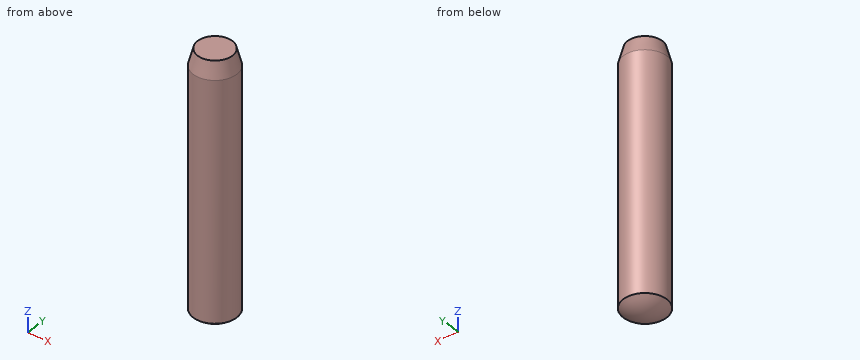
```python
from build123d import *

# Parameters (mm, degrees)
CROQUIS1_R              = 2
SALIENTE_EXTRUIR1_DEPTH = 24
CHAFL_N1_SIZE           = 1.5
CHAFL_N1_SIZE2          = 0.4


with BuildPart() as part:
    # Croquis1 → Saliente-Extruir1 (new body)
    with BuildSketch(Plane.XY):
        Circle(CROQUIS1_R)
    extrude(amount=SALIENTE_EXTRUIR1_DEPTH)

    # Croquis2 → Cortar-Revolución3 (revolve, cut)
    with BuildSketch(Plane(origin=(0, 0, 0), x_dir=(1, 0, 0), z_dir=(0, 1, 0))):
        with BuildLine():
            Line((-2, -0.75), (-2, 0))
            Line((-2, 0), (-2, 0.2))
            Line((-2, 0.2), (0, 0.2))
            Line((0, 0.2), (0, 0))
            ThreePointArc((0, 0), (-1.068000468, -0.193665418), (-2, -0.75))
        make_face()
    revolve(axis=Axis((0, 0, 24), (0, 0, -1)), mode=Mode.SUBTRACT)

    # Chaflán1
    chafl_n1_edges = [part.edges().sort_by_distance(p)[0] for p in [
        (-2, 0, 24),
    ]]
    chafl_n1_side = [part.faces().sort_by_distance(p)[0] for p in [
        (-2, 0, 12.375),
    ]]
    chamfer(chafl_n1_edges, length=CHAFL_N1_SIZE, length2=CHAFL_N1_SIZE2, reference=chafl_n1_side[0])


solid = part.part
```
Verification items for the finished model (mm, model axes). Round coordinates to 2 decimals unless told otherwise and drop trailing zeros. Write each loop counter-clockwise with the first axis right and the second up, starting at its lowest first coordinate (ties: lowest second). Pieces come first, ordered by that corner, then holes. Notation, with made-up numbers: (88.5, -34) -> (126.5, -34) arc R16 cw to (126.5, -5) -> close; hole circle Ø10 at (-14.75, 75). An arc over 180 degrees is marked (long way). Write each question's results on one line, items separated by ' | '. Start each with the question number.
1. Material ranges on probe 1 along Z at (x, y) = (-0.05, 0.05); probe 2 along X at (y, z) = (-1.45, 8.25); probe 3 along X at (y, z) = (-0.3, 3.5), recorded low to high. Write a range as from..to.
2. Depth check by flat-ended pin: P1, Ø2, axis at y = -1, z = 17.5, coming from the -X side; P2, Ø1.5, axis at x = -1, y = 0, coming from the -Z side. Enter the tip coordinate at first touch or a pass-through.
3. Cross-section at A-A (y = 0). Enter the section's corners in (x, z), then the cut area to 3 significant figures.
4. Cross-section at C-C (z = 10). Enter the section's corners in (x, y).
Solutions:
1) probe 1: z = 0..24 | probe 2: x = -1.38..1.38 | probe 3: x = -1.98..1.98
2) P1: stops at x = -2 | P2: stops at z = 0.01
3) outline: (-2, 0.75) arc R3.04 ccw to (2, 0.75) -> (2, 22.5) -> (1.6, 24) -> (-1.6, 24) -> (-2, 22.5) -> close | area: 94.5 mm2
4) outline: circle Ø4 at (0, 0)
